Autodesk Inventor part; units mm, degrees
ref_plane "YZ Plane" through (0, 0, 0) normal (1, 0, 0) x (0, 1, 0)
ref_plane "XZ Plane" through (0, 0, 0) normal (0, 1, 0) x (-1, 0, 0)
ref_plane "XY Plane" through (0, 0, 0) normal (0, 0, 1) x (1, 0, 0)
sketch "Boceto1" plane through (0, 0, 0) normal (0, 1, 0) x (-1, 0, 0)
  circle A0 centre (0, 0) radius 4.5
  dimension "d0" = 9
extrude "Extrusión1" add sketch "Boceto1" along normal blind 1.6
sketch "Boceto2" plane through (0, 1.6, 0) normal (0, 1, 0) x (1, 0, 0)
  circle A0 centre (0, 0) radius 2.5
  dimension "d3" = 5
extrude "Extrusión2" add sketch "Boceto2" along normal blind 12
fillet "Empalme1" radius 0.4 1 edges at (4.5, 0, 0)
fillet "Empalme2" radius 0.2 1 edges at (4.5, 1.6, 0)
sketch "Boceto3" plane through (0, 0, 0) normal (0, -1, 0) x (1, 0, 0)
  line L0 (-1.7321, 0) -> (-0.866, 1.5)
  line L1 (-0.866, 1.5) -> (0.866, 1.5)
  line L2 (0.866, 1.5) -> (1.7321, 0)
  line L3 (1.7321, 0) -> (0.866, -1.5)
  line L4 (0.866, -1.5) -> (-0.866, -1.5)
  line L5 (-0.866, -1.5) -> (-1.7321, 0)
  point P0 (0, 0)
  point P1 (0, 0)
  dimension "d8" = 3
extrude "Extrusión3" cut sketch "Boceto3" against normal blind 2.5
chamfer "Chaflán1" distance 0.5 angle 45 1 edges at (-2.5, 13.6, 0)
thread "Rosca2"
properties part number "Perno M5x8 cabeza plana" material "Hierro, gris"
The model under review builds one solid part; all positions refer to its coordinate system, in mm. A direction names the side the tool comes from. Round coordinates to 2 decimals unless told otherwise and drop trailing zeros. Write each loop counter-clockwise with the first axis right and the second up, starting at its lowest first coordinate (ties: lowest second). Pieces come first, ordered by that corner, then holes. Notation, with made-up numbers: (83.25, 81.5) - (106.25, 81.5) arc R12 ccw to (106.25, 89.5) - close; hole circle Ø7 at (9, -9.75). An arc over 180 degrees is marked (long way). One line per item, written item: value. Start each with the question number.
1. To check wall thickness, follow L1, parallel to X at y = 1.75, z = 0.5; L2, parallel to Z at x = -0.5, y = 1.5; L3, parallel to Y at x = -2, z = 2. State the ranges of each line that lie inside material, in increasing order. Write a range as from..to.
2. Consider section A-A on x = 0. Write out the cut boundary in (y, z).
3. The part is to be moulded in two halves that separate along Y. For faces 1 (the face through (0, 0, -2)), 2 (the face through (-2, 1.6, -2)), 3 (the face through (-0.54, 7.27, -2.44)), say which applies: released by +Y, released by -Y, zero draft, split by the parting line, or undercut.
4. Consider section B-B on y = 12. Write out the cut boundary in (x, z), and give its area (3 significant figures).
5. Machinability: for faces 4 (the face through (0.59, 0.89, -4.46)), 5 (the face through (1.293, 1.232, 0.76)), which of the approach directions +Z, -Z, +X, -X, +Y, -Y give a long, thin tool a straight path to every point of the face, cutting with its end or side? Answer none if there is none.
6. Clearance check with flat-ended pins moving along their axes: P1, Ø3, axis at y = 6.5, z = 1.5, coming from the +X side; P2, Ø3, axis at x = -1, y = 3.5, coming from the +Z side; P3, Ø3, axis at y = 6, z = -1.5, coming from the -X side; P4, Ø1.5, axis at y = 7.5, z = -3.5, coming from the +X side. State where each tip first meets the part, or that it passes through.
Checks:
1. L1: x = -2.45..-1.44, 1.44..2.45
1. L2: z = -4.45..-1.5, 1.5..4.45
1. L3: y = 0..1.6
2. outline: (0, -4.1) arc R0.4 ccw to (0.4, -4.5) - (1.4, -4.5) arc R0.2 ccw to (1.6, -4.3) - (1.6, -2.5) - (13.1, -2.5) - (13.6, -2) - (13.6, 2) - (13.1, 2.5) - (1.6, 2.5) - (1.6, 4.3) arc R0.2 ccw to (1.4, 4.5) - (0.4, 4.5) arc R0.4 ccw to (0, 4.1) - (0, 1.5) - (2.5, 1.5) - (2.5, -1.5) - (0, -1.5) - close
3. face 1: released by -Y
3. face 2: released by +Y
3. face 3: zero draft
4. outline: circle Ø5 at (0, 0)
4. area: 19.6 mm^2
5. face 4: +Y, -Y
5. face 5: -Y
6. P1: stops at x = 2.5
6. P2: stops at z = 2.5
6. P3: stops at x = -2.5
6. P4: passes through
